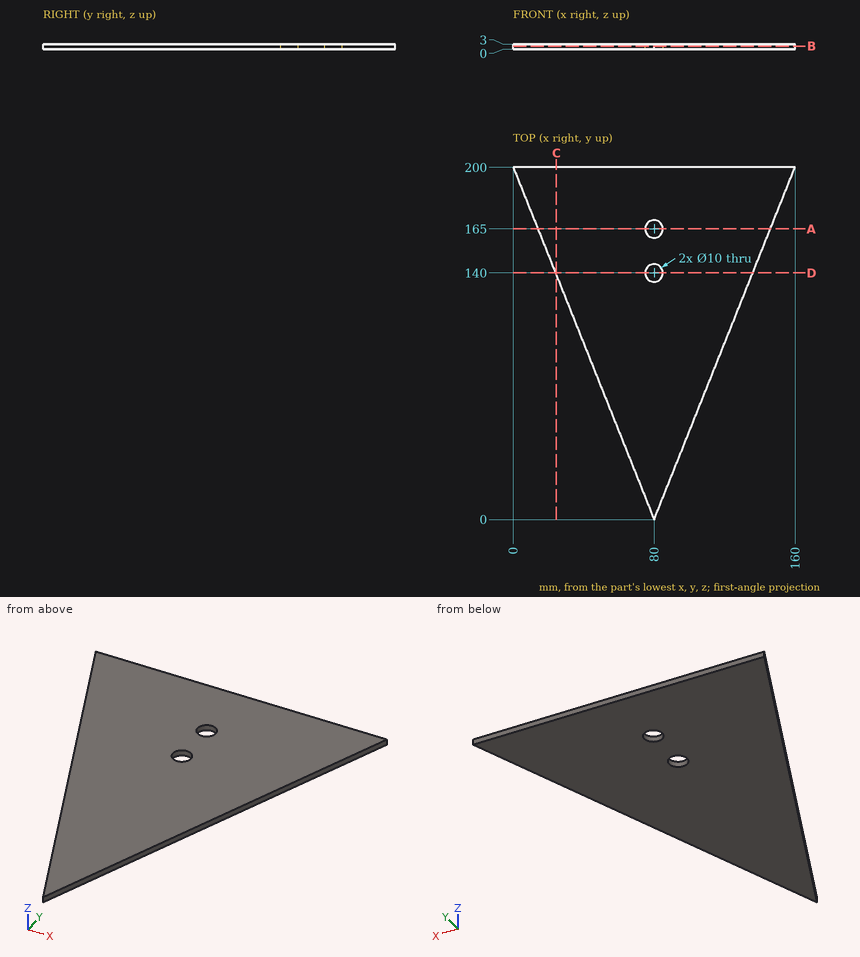
Study the drawing (mm; zero at the part's minimum x, y, z) and answer. Round coordinates to 2 decimals unless told otherwise and drop trailing zeros. Loops run counter-clockwise (first coordinate to the right, second up) from the corner with the lowest first, then second, coordinate; pieces in that order, holes last. Notation, with made-up numbers: M 21,67.25 L 34,67.25 A18 cw 34,71.25 Z; hole C 40.5,4.25 d7. An arc over 180 degrees is marked long. One line per question, with ' | ' between items.
Q1. Each of these flat-tipped pins is pushed along its axis until it touches: pin 1 Ø1.5 at (y, z) = (111, 2) entering from -X; pin 2 Ø1.5 at (x, z) = (20.5, 2) entering from -Y (3 decimals). Where does it stop, or does it pass through?
Conclusion:
pin 1: stops at x = 35.3 | pin 2: stops at y = 146.875
Q2. Consider line 1 along X through (y, z) = (14, 2.85); line 2 along X through (y, z) = (161, 1.5); line 3 along X through (y, z) = (71, 2.8). Determine where each line is inside the solid, lowest interval first. Write a range as from..to.
Conclusion:
line 1: x = 74.4..85.6 | line 2: x = 15.6..77, 83..144.4 | line 3: x = 51.6..108.4
Q3. Find section A-A, the plane y = 165. Give the vertices of the cut face in (x, z).
Conclusion:
outline: M 14,0 L 75,0 L 75,3 L 14,3 Z; M 85,0 L 146,0 L 146,3 L 85,3 Z
Q4. Find section D-D, the plane y = 140. Give the vertices of the cut face in (x, z).
Conclusion:
outline: M 24,0 L 75,0 L 75,3 L 24,3 Z; M 85,0 L 136,0 L 136,3 L 85,3 Z
Q5. Find section C-C, the plane x = 24.5. Give the vertices of the cut face in (y, z), then the cut area to 3 significant figures.
Conclusion:
outline: M 138.75,0 L 200,0 L 200,3 L 138.75,3 Z | area: 184 mm2
Q6. Find section B-B, the plane z = 1.85. Give the vertices of the cut face in (x, y).
Conclusion:
outline: M 0,200 L 80,0 L 160,200 Z; hole C 80,140 d10; hole C 80,165 d10
